For this review, take the finished solid that the model builds, in its own axes (mm). A direction names the side the tool comes from. Coordinates: 2 decimals unless noted, no trailing zeros. Loops run counter-clockwise (first coordinate to the right, second up) from the corner with the lowest first, then second, coordinate; pieces in that order, holes last. Notation, with made-up numbers: M -13.75,25 L 6.25,25 A28 ccw 6.25,45 Z; hole C 26,76.5 d3. An arc over 180 degrees is marked long. Answer as a JSON object with one key per item and string values. Group by question number.
Item 1: Wall thickness on L1, parallel to Y at x = 115, z = -1; L2, parallel to Z at x = 107, y = 15.5 (3 decimals); L3, parallel to Y at x = 9.5, z = -0.9: over which ranges is each line inside the solid? List them lowest first. Write a range as from..to.
Item 2: Add section C-C (y = 54). State the section outline as (x, z) points (3 decimals), then the cut area to 4 significant figures.
Item 3: Insertion check: pin 1 (5 mm diameter, centred on x = 9, z = 66.825, fed in from +Y); pin 2 (14.5 mm diameter, centred on x = 8.5, z = 32, fed in from -Y); pin 3 (1.5 mm diameter, centred on x = 101.5, y = 16.5, fed in from +Z); pin 4 (2.5 mm diameter, centred on x = 66.5, z = -2, fed in from +Y). Each pin has a flat end and moves straight along its axis. Give the tip position at first contact, or say it passes through.
Item 4: Add section B-B (x = 9.5). State the section outline as (y, z) points (3 decimals).
Item 5: Tool access review of faces 1 (the face through (72, 18, -2)), 2 (the face through (6.9, 76.57, 68.44)), 3 (the face through (9, 75, 39)): name each direction out of +Z, -Z, +X, -X, +Y, -Y from which nothing blocks a thin tool from reaching the whole face with its end or side.
Item 6: Add section A-A (x = 115.5). State the section outline as (y, z) points (3 decimals).
Item 7: Mouldability with a two-part tool opening along Y and no side actions: class faces 4 (the face through (113.497, 9.631, -1.61)), 5 (the face through (9, 78.175, 38)), 6 (the face through (125, 9, -2)) as +Y half, -Y half, draft (parallel to the pull), parting line (faces both ways), or undercut.
Item 8: Add section D-D (z = 2.5). State the section outline as (x, y) points (3 decimals).
from build123d import *

# Parameters (mm, degrees)
BASE_FLANGE1_DEPTH           = 3.175
EDGE_FLANGE1_STRIP_W         = 14.1732
EDGE_FLANGE1_STRIP_H         = 3.175
EDGE_FLANGE1_STRIP_CUT_DEPTH = 18
EDGE_FLANGE1_DEPTH           = 18
M5X0_8_TAPPED_HOLE1_D        = 4.2
HOLE2_START                  = 75
HOLE2_OUTLINE_R              = 2.65
HOLE2_DEPTH                  = 3.175


# Read off the part's stored shape, not the designer's step: Hole2
# Sheet-metal steps are written as plain solids
with BuildPart() as part:
    # Sketch1 → Base-Flange1 (new body)
    with BuildSketch(Plane.XY):
        Polygon((0, 75), (0, 0), (125, 0), (125, 18), (18, 18), (18, 75), align=None)
    extrude(amount=-BASE_FLANGE1_DEPTH)

    # Edge-Flange1 strip (across the edge) → Edge-Flange1 strip cut (cut)
    with BuildSketch(Plane(origin=(18, 75, 0), x_dir=(0, -1, 0), z_dir=(-1, 0, 0))):
        with Locations((-6.35, -1.5875)):
            Rectangle(EDGE_FLANGE1_STRIP_W, EDGE_FLANGE1_STRIP_H)
    extrude(amount=EDGE_FLANGE1_STRIP_CUT_DEPTH, mode=Mode.SUBTRACT)

    # Edge-Flange1 section (across the edge) → Edge-Flange1 (add)
    with BuildSketch(Plane(origin=(18, 75, 0), x_dir=(0, -1, 0), z_dir=(-1, 0, 0))):
        with BuildLine():
            Line((-3.175, 0.7366), (-3.175, 76.825))
            Line((-3.175, 76.825), (0, 76.825))
            Line((0, 76.825), (0, 0.7366))
            ThreePointArc((0, 0.7366), (0.215745145, 0.215745145), (0.7366, 0))
            Line((0.7366, 0), (0.7366, -3.175))
            ThreePointArc((0.7366, -3.175), (-2.029318885, -2.029318885), (-3.175, 0.7366))
        make_face()
    extrude(amount=EDGE_FLANGE1_DEPTH)

    # M5x0.8 Tapped Hole1 (through all)
    with Locations(Plane.XY):
        with Locations((9.5, 9), (115.5, 9)):
            Hole(M5X0_8_TAPPED_HOLE1_D / 2)

    # Hole2 outline → Hole2 (cut)
    with BuildSketch(Plane(origin=(0, 0, 0), x_dir=(1, 0, 0), z_dir=(0, 1, 0)).offset(HOLE2_START)):
        with Locations((9, -66.825)):
            Circle(HOLE2_OUTLINE_R)
    extrude(amount=HOLE2_DEPTH, mode=Mode.SUBTRACT)


solid = part.part
From the geometry:
{
 "1": {"L1": "y = 0..6.96, 11.04..18", "L2": "z = -3.175..0", "L3": "y = 0..6.9, 11.1..77.82"},
 "2": {"outline": "M 0,-3.175 L 18,-3.175 L 18,0 L 0,0 Z", "area": "57.15 mm²"},
 "3": {"pin 1": "passes through", "pin 2": "stops at y = 75", "pin 3": "stops at z = 0", "pin 4": "stops at y = 18"},
 "4": {"outline": "M 0,-3.175 L 6.9,-3.175 L 6.9,0 L 0,0 Z; M 11.1,-3.175 L 74.263,-3.175 A3.912 ccw 78.175,0.737 L 78.175,64.223 L 75,64.223 L 75,0.737 A0.737 cw 74.263,0 L 11.1,0 Z; M 75,69.427 L 78.175,69.427 L 78.175,76.825 L 75,76.825 Z"},
 "5": {"face 1": "+Z, -Z, +X, +Y", "face 2": "+Y, -Y", "face 3": "+Z, +X, -X, -Y"},
 "6": {"outline": "M 0,-3.175 L 6.9,-3.175 L 6.9,0 L 0,0 Z; M 11.1,-3.175 L 18,-3.175 L 18,0 L 11.1,0 Z"},
 "7": {"face 4": "undercut", "face 5": "+Y half", "face 6": "draft"},
 "8": {"outline": "M 0,75 L 18,75 L 18,78.175 L 0,78.175 Z"}
}
